Autodesk Fusion 360 part; units mm, degrees
sketch "Sketch1" plane through (0, 0, 0) normal (0, 1, 0) x (1, 0, 0)
  line L0 (0, 0) -> (-70, 0)
  line L1 (-70, 0) -> (-70, 70)
  line L2 (-70, 70) -> (0, 70)
  line L3 (0, 70) -> (0, 0)
  dimension "d1" = 70
  dimension "d2" = 70
extrude "Extrude1" add sketch "Sketch1" along normal blind 2
sketch "Sketch2" plane through (0, 2, 0) normal (0, 1, 0) x (-1, 0, 0)
  line L0 (0, -70) -> (70, -70)
  line L1 (70, -70) -> (70, 0)
  line L2 (70, 0) -> (0, 0)
  line L3 (0, 0) -> (0, -70)
  circle A0 centre (2.7499, -2.7499) radius 1.5
  line L4 (70, -70) -> (73.889, -70) construction
  line L5 (0, -70) -> (3.889, -70) construction
  circle A1 centre (67.2501, -67.2501) radius 1.5
  circle A2 centre (2.7499, -67.2501) radius 1.5
  circle A3 centre (67.2501, -2.7499) radius 1.5
  dimension "d5" = 3.889
  dimension "d6" = 3
  dimension "d7" = 3.889
  dimension "d9" = 3.889
  dimension "d11" = 3.889
  dimension "d12" = 3
  dimension "d13" = 3
  dimension "d14" = 3
extrude "Extrude2" add sketch "Sketch2" along normal blind 20 contours A0 | A1 | A2 | A3
fillet "Fillet1" radius 2 4 edges at (-70, 1, 0) (0, 1, 0) (0, 1, -70) (-70, 1, -70)
sketch "Sketch3" plane through (0, 2, 0) normal (0, 1, 0) x (-1, 0, 0)
  arc A0 (68, -70) -> (70, -68) centre (68, -68) ccw
  line L0 (70, -68) -> (70, -2)
  arc A1 (70, -2) -> (68, 0) centre (68, -2) ccw
  line L1 (68, 0) -> (2, 0)
  arc A2 (2, 0) -> (0, -2) centre (2, -2) ccw
  line L2 (0, -2) -> (0, -68)
  arc A3 (0, -68) -> (2, -70) centre (2, -68) ccw
  line L3 (2, -70) -> (68, -70)
  circle A4 centre (67.2501, -2.7499) radius 1.5
  circle A5 centre (67.2501, -67.2501) radius 1.5
  circle A6 centre (2.7499, -2.7499) radius 1.5
  circle A7 centre (2.7499, -67.2501) radius 1.5
  line L4 (0, 0) -> (70, 0)
  line L5 (70, 0) -> (70, -70)
  line L6 (70, -70) -> (0, -70)
  line L7 (0, -70) -> (0, 0)
  line L8 (68.0791, -66) -> (68, -66)
  line L9 (36, -1.414) -> (5.414, -1.414)
  line L10 (2, -5.414) -> (5.414, -5.414)
  line L11 (5.414, -5.414) -> (5.414, -1.414)
  line L12 (2, -5.414) -> (1.414, -5.414)
  line L13 (1.414, -15) -> (1.414, -5.414)
  line L14 (1.414, -15) -> (1.414, -64.586)
  line L15 (1.414, -64.586) -> (5.414, -64.586)
  line L16 (5.414, -64.586) -> (5.414, -68.586)
  line L17 (32, -68.586) -> (5.414, -68.586)
  line L18 (32, -68.586) -> (64.586, -68.586)
  line L19 (64.586, -68.586) -> (64.586, -64.586)
  line L20 (64.586, -64.586) -> (68.586, -64.586)
  line L21 (36, -1.414) -> (64.586, -1.414)
  line L22 (64.586, -1.414) -> (64.586, -5.414)
  line L23 (68.586, -24) -> (68.586, -5.414)
  line L24 (64.586, -5.414) -> (68.586, -5.414)
  line L25 (68.586, -24) -> (68.586, -64.586)
  line L26 (68, -66) -> (68, -65.951)
  dimension "d22" = 5.414
  dimension "d29" = 90
extrude "Extrude3" add sketch "Sketch3" along normal blind 10 contours A0 L0 A1 L1 A2 L2 A3 L3 L4 L5 L6 L7
fillet "Fillet2" radius 2 2 edges at (-5.414, 7, -64.586) (-64.586, 7, -64.586)
fillet "Fillet3" radius 2 2 edges at (-64.586, 7, -5.414) (-5.414, 7, -5.414)
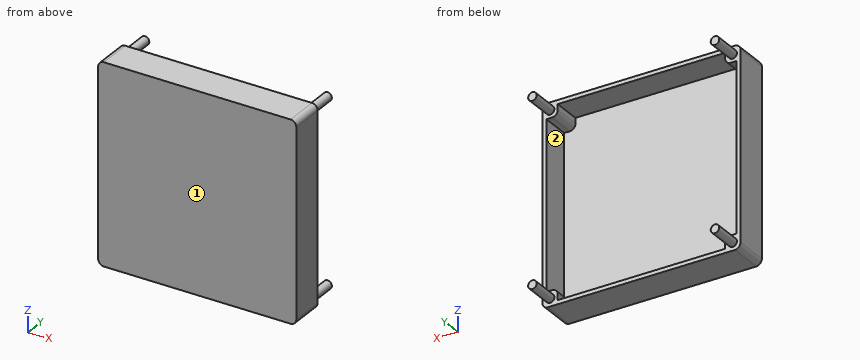
Verification items for the finished model (mm, model axes). Face numbers are marked on the shaded views. A direction names the side the tool comes from. Round coordinates to 2 decimals unless told otherwise and drop trailing zeros. Write each loop counter-clockwise with the first axis right and the second up, starting at its lowest first coordinate (ties: lowest second). Pieces come first, ordered by that corner, then holes. Notation, with made-up numbers: (-6.5, -0.5) - (22.5, -0.5) arc R30 ccw to (22.5, 36.5) - close; hole circle Ø4 at (-35, -0.5). An arc over 180 degrees is marked (long way). Answer as a JSON object with one key per item and string values. Group by question number.
Q1. Go/stop test with a flat-tipped pin: pin 1 Ø20 at (x, z) = (-27.5, -45) entering from +Y. Record where the tip stops, or that it passes through.
Q2. Section check D-D, the plane y = 13.25. Enter the section's corners in (x, z).
Q3. Section check C-C, the plane z = -42.5. Enter the section's corners in (x, y), plus the area to 3 significant figures.
Q4. Section check B-B, the plane x = -9. Enter the section's corners in (y, z).
Q5. Section check A-A, the plane y = 4.75. Enter the section's corners in (x, z).
Q6. Thickness scan on line 1 (Z direction, x = -7, y = 7.25); line 2 (Y direction, x = -20, z = -32). Record the ranges inside material, lowest first.
Q7. Tool access check on the marked faces 1 and 2. Record the directions out of +Z, -Z, +X, -X, +Y, -Y that give a thin tool (end or side, any length) a straight path to the whole face; none if there is none.
Found:
{
 "1": {"pin 1": "stops at y = 2"},
 "2": {"outline": "circle Ø3 at (-67.25, -67.25); circle Ø3 at (-67.25, -2.75); circle Ø3 at (-2.75, -67.25); circle Ø3 at (-2.75, -2.75)"},
 "3": {"outline": "(-70, 0) - (0, 0) - (0, 12) - (-1.41, 12) - (-1.41, 2) - (-68.59, 2) - (-68.59, 12) - (-70, 12) - close", "area": "168 mm^2"},
 "4": {"outline": "(0, -70) - (12, -70) - (12, -68.59) - (2, -68.59) - (2, -1.41) - (12, -1.41) - (12, 0) - (0, 0) - close"},
 "5": {"outline": "(-70, -68) arc R2 ccw to (-68, -70) - (-2, -70) arc R2 ccw to (0, -68) - (0, -2) arc R2 ccw to (-2, 0) - (-68, 0) arc R2 ccw to (-70, -2) - close; hole (-68.59, -64.59) - (-66.59, -64.59) arc R2 cw to (-64.59, -66.59) - (-64.59, -68.59) - (-5.41, -68.59) - (-5.41, -66.59) arc R2 cw to (-3.41, -64.59) - (-1.41, -64.59) - (-1.41, -5.41) - (-3.41, -5.41) arc R2 cw to (-5.41, -3.41) - (-5.41, -1.41) - (-64.59, -1.41) - (-64.59, -3.41) arc R2 cw to (-66.59, -5.41) - (-68.59, -5.41) - close"},
 "6": {"line 1": "z = -70 to -68.59, -1.41 to 0", "line 2": "y = 0 to 2"},
 "7": {"face 1": "+Z, -Z, +X, -X, -Y", "face 2": "+Y"}
}
